Read the model definition and answer for the solid it produces. Units are mm, in the model's axes. Face numbers are marked on the shaded views. A direction names the side the tool comes from. Give positions to 0.01 mm unless a question says otherwise; leave off trailing zeros. Order: outer loops, then holes, each group sorted by start corner. A loop starts at its lowest first (then second) coordinate and runs counter-clockwise, first axis right, second up. Notation, with made-up numbers: (62, -16) -> (76, -16) arc R18 cw to (76, -1) -> close; hole circle Ø8 at (41.25, 0). An arc over 180 degrees is marked (long way). Use one line per item in the form item = value.
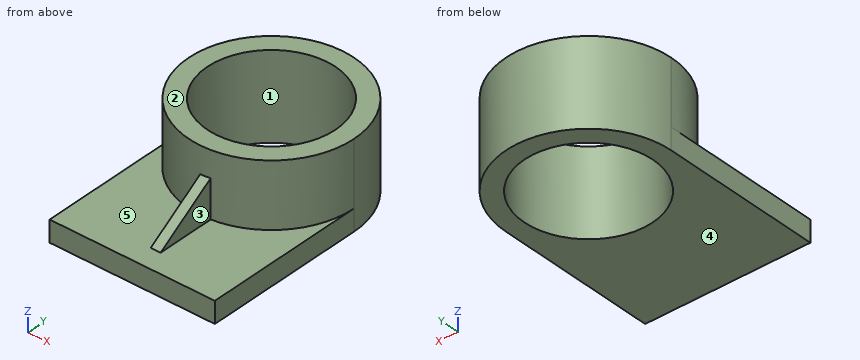
```python
from build123d import *

# Parameters (mm, degrees)
F1_DEPTH = 12.7
F3_DEPTH = 50.8
F4_R     = 38.0054760492
F5_DEPTH = 50.801
F9_DEPTH = 5.842


with BuildPart() as f1:
    # F0 (on Top) → F1 (new body)
    with BuildSketch(Plane.XY):
        with BuildLine():
            Line((-49.0042343736, -47.9455031455), (49.0042343736, -47.9455031455))
            Line((49.0042343736, -47.9455031455), (49.0042343736, 47.9455031455))
            ThreePointArc((49.0042343736, 47.9455031455), (0, -1.0587312281), (-49.0042343736, 47.9455031455))
            Line((-49.0042343736, 47.9455031455), (-49.0042343736, -47.9455031455))
        make_face()
    extrude(amount=F1_DEPTH)

    # F2 (on Top) → F3 (join)
    with BuildSketch(Plane.XY):
        with BuildLine():
            ThreePointArc((-49.0042343736, 47.9455031455), (0, -1.0587312281), (49.0042343736, 47.9455031455))
            ThreePointArc((49.0042343736, 47.9455031455), (0, 96.949737519), (-49.0042343736, 47.9455031455))
        make_face()
    extrude(amount=F3_DEPTH)

    # F4 (on face) → F5 (cut, through all)
    with BuildSketch(Plane.XY.offset(50.8)):
        with Locations((0, 47.9455031455)):
            Circle(F4_R)
    extrude(amount=-F5_DEPTH, mode=Mode.SUBTRACT)

    # F8 (on plane+point) → F9 (join)
    with BuildSketch(Plane.YZ):
        Polygon((0, 35.7907004654), (-35.212572664, 12.7), (0, 12.7), align=None)
    extrude(amount=F9_DEPTH)


solid = f1.part
```
Item 1: The part is cut by section D-D on y = 3.5. Give the vertices of the cut face in (x, z).
Checks:
outline = (-49, 0) -> (49, 0) -> (49, 12.7) -> (20.64, 12.7) -> (20.64, 50.8) -> (-20.64, 50.8) -> (-20.64, 12.7) -> (-49, 12.7) -> close
Item 2: Given pin 1 Ø18 at (y, z) = (-23, 22) entering from -X; pin 2 Ø7 at (y, z) = (-23, 23.5) entering from +X; pin 3 Ø3 at (x, z) = (-35.5, 24.5) entering from +Y, each flat-ended and moving along its own axis, determine where each tip first touches the part or whether it passes through.
Checks:
pin_1 = 0
pin_2 = 5.84
pin_3 = 83.24
Item 3: Straight lines are drawn through the part: L1, parallel to Y at x = 0, z = 11; L2, parallel to Z at x = 22, y = -20; L3, parallel to Y at x = 7.5, z = 14. For each, find the intervals that lie inside material, in ascending order. Write a range as from..to.
Checks:
L1 = -47.95..9.94, 85.95..96.95
L2 = 0..12.7
L3 = -0.48..10.69, 85.2..96.37
Item 4: The part is cut by section A-A on y = 36. Give the vertices of the cut face in (x, z), and give its area (3 significant figures).
Checks:
outline = (-49, 0) -> (-36.08, 0) -> (-36.08, 50.8) -> (-47.53, 50.8) -> (-47.53, 12.7) -> (-49, 12.7) -> close; (36.08, 0) -> (49, 0) -> (49, 12.7) -> (47.53, 12.7) -> (47.53, 50.8) -> (36.08, 50.8) -> close
area = 1,200 mm²
Item 5: Determine the mould class of the marked faces 1, 2 and 3 for opening direction X: +X half, -X half, draft (parallel to the pull), parting line (faces both ways), or undercut.
Checks:
face_1 = undercut
face_2 = draft
face_3 = +X half
Item 6: The part is cut by section C-C on z = 30. Give the vertices of the cut face in (x, y), and give its area (3 significant figures).
Checks:
outline = (0, -8.83) -> (5.84, -8.83) -> (5.84, -0.71) arc R49 ccw (long way) to (0, -1.06) -> close; hole circle Ø76.01 at (0, 47.95)
area = 3,050 mm²
Item 7: Which of the six approach directions +Z, -Z, +X, -X, +Y, -Y give full straight-line access (tool end or side, diameter ignored) to the marked faces 4 and 5?
Checks:
face_4 = -Z, +X, -X, +Y, -Y
face_5 = +Z, -Y
Item 8: The part is cut by section B-B on x = -30. Give the vertices of the cut face in (y, z).
Checks:
outline = (-47.95, 0) -> (24.61, 0) -> (24.61, 50.8) -> (9.2, 50.8) -> (9.2, 12.7) -> (-47.95, 12.7) -> close; (71.28, 0) -> (86.69, 0) -> (86.69, 50.8) -> (71.28, 50.8) -> close
